Input: part model. Units: mm. Frame: model coordinates. Face numbers are marked on the shaded views. A direction names the side the tool comes from. Round coordinates to 2 decimals unless told otherwise and drop trailing zeros. Order: outer loops, then holes, each group sorted by start corner. A loop starts at its lowest first (then second) coordinate and runs counter-clockwise, first axis right, second up.
Item 1: Cut plane A-A on z = -7.75. Output: boundary loops of the cut face in (x, y), then the cut area to 3 significant figures.
Item 2: Reachability of the marked faces 1, 2 and 3 from +Z, -Z, +X, -X, +Y, -Y: full face, straight path, thin tool, end or side. Return the list, or none.
Item 3: First-contact query: pin 1 (3.5 mm diameter, centred on x = 84, z = -4.5, fed in from -Y); pin 2 (1 mm diameter, centred on y = -22.5, z = -3, fed in from +X); pin 3 (6 mm diameter, centred on x = -0.5, z = -2, fed in from +Y). Flat tips, straight axial feed; report the tip coordinate or a pass-through.
Item 4: Cut plane C-C on z = 1. Output: boundary loops of the cut face in (x, y).
Item 5: Mould query, pull axis Y, two halves, no side actions, for the marked faces 4, 5 and 6. Classes: released by +Y, released by -Y, zero draft, split by the parting line, or undercut.
Item 6: Cut plane D-D on x = 52. Output: boundary loops of the cut face in (y, z), then the cut area to 3 significant figures.
Item 7: Line query: L1, parallel to Y at x = 69, z = -4.5; L2, parallel to X at y = -18, z = -5.75; L3, parallel to X at y = -9, z = -0.5. Output: solid intervals per line, ascending.
Item 8: Cut plane B-B on y = 2. Output: boundary loops of the cut face in (x, z), then the cut area to 3 significant figures.
Autodesk Fusion 360 part; units mm, degrees
sketch "Sketch1" plane through (0, 0, 0) normal (0, 0, 1) x (1, 0, 0) in component "Exercise 2"
  circle A0 centre (0, 0) radius 30
  line L0 (30, 0) -> (109, 0) construction
  circle A1 centre (129, 0) radius 20
  line L1 (-23.094, 0) -> (-11.547, -20)
  line L2 (-11.547, -20) -> (11.547, -20)
  line L3 (11.547, -20) -> (23.094, 0)
  line L4 (23.094, 0) -> (11.547, 20)
  line L5 (11.547, 20) -> (-11.547, 20)
  line L6 (-11.547, 20) -> (-23.094, 0)
  line L7 (129, 15) -> (114.7342, 4.6353)
  line L8 (114.7342, 4.6353) -> (120.1832, -12.1353)
  line L9 (120.1832, -12.1353) -> (137.8168, -12.1353)
  line L10 (137.8168, -12.1353) -> (143.2658, 4.6353)
  line L11 (143.2658, 4.6353) -> (129, 15)
  line L12 (28.2843, 10) -> (111.6795, 10)
  line L13 (28.2843, -10) -> (111.6795, -10)
  line L14 (41.522, 10) -> (41.522, -10) construction
  line L15 (41.522, 0) -> (50, 0) construction
  line L16 (69.5, 0) -> (69.5, 26.8283) construction
  line L17 (99.5, 5) -> (39.5, 5)
  line L18 (39.5, -5) -> (99.5, -5)
  line L19 (99.5, 5) -> (39.5, -5) construction
  line L20 (39.5, 5) -> (99.5, -5) construction
  arc A2 (41.522, 4.5729) -> (41.522, -4.5729) centre (39.5, 0) ccw
  arc A3 (97.8784, -4.7297) -> (97.8784, 4.7297) centre (99.5, 0) ccw
  point P0 (129, 0)
  point P1 (69.5, 0)
  dimension "d13" = 60
  dimension "d14" = 129
  dimension "d15" = 40
  dimension "d17" = 20
  dimension "d18" = 15
  dimension "d19" = 20
  dimension "d20" = 60
  dimension "d21" = 10
  dimension "d22" = 10
extrude "Extrude1" add sketch "Sketch1" along normal mid plane 20 contours A0 | A1 makes body 1 at (27.1662, -12.7278, 3.3333) makes body 2 at (148.9006, -1.9914, -3.3333) in component "Exercise 2"
extrude "Extrude2" add sketch "Sketch1" along normal mid plane 12 contours A0 A1 L12 L13 bodies 1 2 in component "Exercise 2"
extrude "Extrude3" add sketch "Sketch1" along normal mid plane 6 contours L17 L18 A2 A3 bodies 1 in component "Exercise 2"
component "Exercise 2" placed x (1, 0, 0) y (0, 1, 0) z (0, 0, 1) at (0, 0, 0)
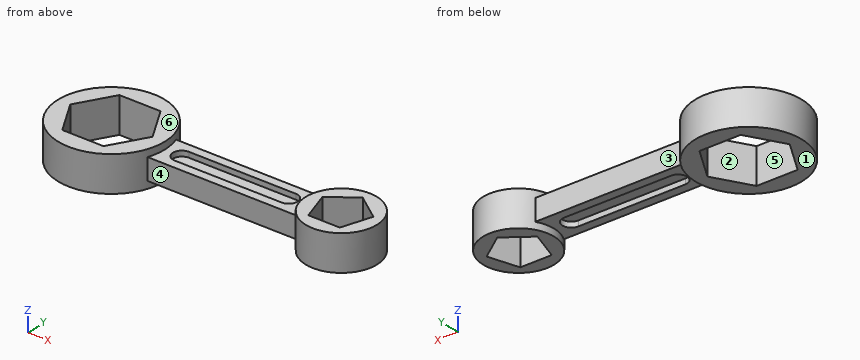
From the geometry:
1. outline: circle Ø60 at (0, 0); circle Ø40 at (129, 0); hole (-23.09, 0) - (-11.55, -20) - (11.55, -20) - (23.09, 0) - (11.55, 20) - (-11.55, 20) - close; hole (114.73, 4.64) - (120.18, -12.14) - (137.82, -12.14) - (143.27, 4.64) - (129, 15) - close
1. area: 2,160 mm2
2. face 1: -Z, +X, -X, +Y, -Y
2. face 2: +Z, -Z
2. face 3: +Z, -Z, +Y
3. pin 1: stops at y = -10
3. pin 2: stops at x = 20.4
3. pin 3: stops at y = 30
4. outline: (28.28, -10) - (111.68, -10) arc R20 ccw (long way) to (111.68, 10) - (28.28, 10) arc R30 ccw (long way) to start; hole (-23.09, 0) - (-11.55, -20) - (11.55, -20) - (23.09, 0) - (11.55, 20) - (-11.55, 20) - close; hole (114.73, 4.64) - (120.18, -12.14) - (137.82, -12.14) - (143.27, 4.64) - (129, 15) - close
5. face 4: released by -Y
5. face 5: undercut
5. face 6: zero draft
6. outline: (-10, -6) - (-5, -6) - (-5, -3) - (5, -3) - (5, -6) - (10, -6) - (10, 6) - (5, 6) - (5, 3) - (-5, 3) - (-5, 6) - (-10, 6) - close
6. area: 180 mm2
7. L1: y = -10 to -5, 5 to 10
7. L2: x = -24 to -12.7, 12.7 to 24, 120.28 to 137.72
7. L3: x = -28.62 to -17.9, 17.9 to 119.16, 138.84 to 146.86
8. outline: (-29.93, -10) - (-21.94, -10) - (-21.94, 10) - (-29.93, 10) - close; (21.94, -10) - (29.93, -10) - (29.93, -6) - (34.92, -6) - (34.92, -3) - (104.08, -3) - (104.08, -6) - (109.1, -6) - (109.1, -10) - (115.59, -10) - (115.59, 10) - (109.1, 10) - (109.1, 6) - (104.08, 6) - (104.08, 3) - (34.92, 3) - (34.92, 6) - (29.93, 6) - (29.93, 10) - (21.94, 10) - close; (142.41, -10) - (148.9, -10) - (148.9, 10) - (142.41, 10) - close
8. area: 1,110 mm2
